from build123d import *

# Parameters (mm, degrees)
SKETCH1_W           = 45
SKETCH1_H           = 19.5
BOSS_EXTRUDE1_DEPTH = 2.5
SKETCH2_W           = 5
SKETCH2_H           = 19.5
BOSS_EXTRUDE2_DEPTH = 4
FILLET1_R           = 0.5
CHAMFER1_SIZE       = 0.5
CHAMFER1_SIZE2      = 5.715026151


with BuildPart() as part:
    # Sketch1 → Boss-Extrude1 (new body)
    with BuildSketch(Plane(origin=(0, 0, 0), x_dir=(1, 0, 0), z_dir=(0, 1, 0))):
        with Locations((1.28516624, -1.137468031)):
            Rectangle(SKETCH1_W, SKETCH1_H)
    extrude(amount=BOSS_EXTRUDE1_DEPTH)

    # Sketch2 → Boss-Extrude2 (add)
    with BuildSketch(Plane(origin=(0, 2.5, 0), x_dir=(1, 0, 0), z_dir=(0, 1, 0))):
        with Locations((21.28516624, -1.137468031)):
            Rectangle(SKETCH2_W, SKETCH2_H)
    extrude(amount=BOSS_EXTRUDE2_DEPTH)

    # Fillet1
    fillet1_edges = [part.edges().sort_by_distance(p)[0] for p in [
        (23.78516624, 6.5, 1.137468031),
        (18.78516624, 6.5, 1.137468031),
    ]]
    fillet(fillet1_edges, radius=FILLET1_R)

    # Chamfer1
    chamfer1_edges = [part.edges().sort_by_distance(p)[0] for p in [
        (-21.21483376, 2.5, 1.137468031),
    ]]
    chamfer1_side = [part.faces().sort_by_distance(p)[0] for p in [
        (-21.21483376, 1.25, 1.137468031),
    ]]
    chamfer(chamfer1_edges, length=CHAMFER1_SIZE, length2=CHAMFER1_SIZE2, reference=chamfer1_side[0])


solid = part.part
The listing builds one solid part. Answer for the finished solid, in the listing's coordinates (mm). A direction names the side the tool comes from. Give positions to 0.01 mm unless a question says otherwise; leave off trailing zeros. Loops run counter-clockwise (first coordinate to the right, second up) from the corner with the lowest first, then second, coordinate; pieces in that order, holes last.
Item 1: A cutting plane is placed at B-B (x = -1.5). Give the vertices of the cut face in (y, z).
Derived:
outline: (0, -8.61) - (2.5, -8.61) - (2.5, 10.89) - (0, 10.89) - close
Item 2: This flat-tipped pin is pushed along its axis until it touches: pin 1 Ø5 at (x, z) = (-7, 9) entering from -Y. Where does it stop, or does it pass through?
Derived:
pin 1: stops at y = 0
Item 3: A cutting plane is placed at C-C (y = 4). Give the vertices of the cut face in (x, z).
Derived:
outline: (18.79, -8.61) - (23.79, -8.61) - (23.79, 10.89) - (18.79, 10.89) - close
Item 4: A cutting plane is placed at A-A (z = 9.5). Give the vertices of the cut face in (x, y), then the cut area to 3 significant figures.
Derived:
outline: (-21.21, 0) - (23.79, 0) - (23.79, 6) arc R0.5 ccw to (23.29, 6.5) - (19.29, 6.5) arc R0.5 ccw to (18.79, 6) - (18.79, 2.5) - (-15.5, 2.5) - (-21.21, 2) - close
area: 131 mm2
Item 5: A tool of negligible diameter and unlimited length cuts with its end or side. For faces 1 (the flat face through (18.785, 4, 1)), 2 (the flat face through (21, 6.5, 1)), from which of +Z, -Z, +X, -X, +Y, -Y can it reach the whole face along a straight path? Write none if from no direction.
Derived:
face 1: +Z, -Z, -X, +Y
face 2: +Z, -Z, +X, -X, +Y
Item 6: Find the intervals of material crossed by line 1 along Y through (x, z) = (11, 0.5); line 2 along X through (y, z) = (4, 9.75); line 3 along Y through (x, z) = (-18.5, 5), in increasing order.
Derived:
line 1: y = 0 to 2.5
line 2: x = 18.79 to 23.79
line 3: y = 0 to 2.24
